Read the model definition and answer for the solid it produces. Units are mm, in the model's axes. Face numbers are marked on the shaded views. Round coordinates to 2 decimals unless told otherwise and drop trailing zeros. Order: outer loops, then holes, each group sorted by start corner. A loop starts at its lowest first (then second) coordinate and runs counter-clockwise, first axis right, second up.
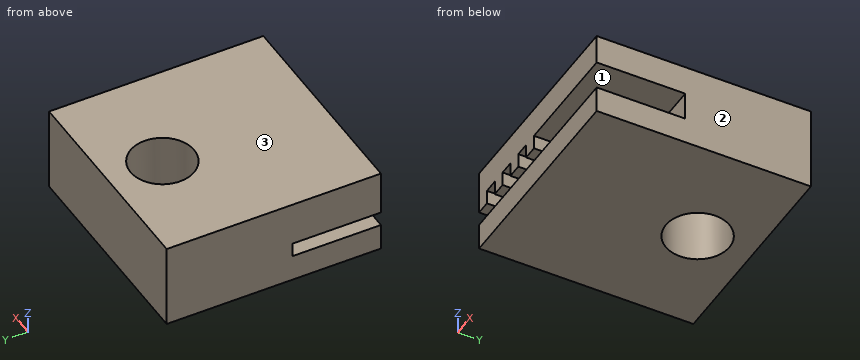
from build123d import *

# Parameters (mm, degrees)
F0_W     = 15
F0_H     = 15
F1_DEPTH = 6
F3_DEPTH = 6.2
F4_R     = 2.223391
F5_DEPTH = 25


with BuildPart() as f1:
    # F0 (on Top) → F1 (new body)
    with BuildSketch(Plane.XY):
        with Locations((13.635715, 2.612354)):
            Rectangle(F0_W, F0_H)
    extrude(amount=F1_DEPTH)

    # F2 (on face) → F3 (cut)
    with BuildSketch(Plane.XZ.offset(4.887646)):
        Polygon((6.135715, 2.883776), (6.135715, 1.883776), (21.135715, 1.883776), (21.135715, 3.883776), (14.135715, 3.883776), (13.135715, 3.883776), (13.135715, 2.883776), (12.135715, 2.883776), (12.135715, 3.883776), (11.135715, 3.883776), (11.135715, 2.883776), (10.135715, 2.883776), (10.135715, 3.883776), (9.135715, 3.883776), (9.135715, 2.883776), (8.135715, 2.883776), (8.135715, 3.883776), (7.135715, 3.883776), (7.135715, 2.883776), align=None)
    extrude(amount=-F3_DEPTH, mode=Mode.SUBTRACT)

    # F4 (on face) → F5 (cut)
    with BuildSketch(Plane(origin=(0, 0, 0), x_dir=(1, 0, 0), z_dir=(0, 0, -1))):
        with Locations((13.635715, -6.298021)):
            Circle(F4_R)
    extrude(amount=-F5_DEPTH, mode=Mode.SUBTRACT)


solid = f1.part
Q1. A cutting plane is placed at C-C, the plane z = 0.8. Give the vertices of the cut face in (x, y), plus the area to 3 significant figures.
Outcome:
outline: (6.14, -4.89) - (21.14, -4.89) - (21.14, 10.11) - (6.14, 10.11) - close; hole circle Ø4.45 at (13.64, 6.3)
area: 209 mm2
Q2. A cutting plane is placed at B-B, the plane x = 9.5. Give the vertices of the cut face in (y, z), plus the area to 3 significant figures.
Outcome:
outline: (-4.89, 0) - (10.11, 0) - (10.11, 6) - (-4.89, 6) - (-4.89, 3.88) - (1.31, 3.88) - (1.31, 1.88) - (-4.89, 1.88) - close
area: 77.6 mm2
Q3. A cutting plane is placed at A-A, the plane y = -1. Give the vertices of the cut face in (x, z).
Outcome:
outline: (6.14, 0) - (21.14, 0) - (21.14, 1.88) - (6.14, 1.88) - close; (6.14, 2.88) - (7.14, 2.88) - (7.14, 3.88) - (8.14, 3.88) - (8.14, 2.88) - (9.14, 2.88) - (9.14, 3.88) - (10.14, 3.88) - (10.14, 2.88) - (11.14, 2.88) - (11.14, 3.88) - (12.14, 3.88) - (12.14, 2.88) - (13.14, 2.88) - (13.14, 3.88) - (21.14, 3.88) - (21.14, 6) - (6.14, 6) - close
Q4. For a pull along Z with two mould halves and no side action, classify the marked faces 1, 2 and 3 as released by +Z, released by -Z, zero draft, split by the parting line, or undercut.
Outcome:
face 1: undercut
face 2: zero draft
face 3: released by +Z
Q5. A cutting plane is placed at D-D, the plane y = 7.75. Give the vertices of the cut face in (x, z), plus the area to 3 significant figures.
Outcome:
outline: (6.14, 0) - (11.95, 0) - (11.95, 6) - (6.14, 6) - close; (15.32, 0) - (21.14, 0) - (21.14, 6) - (15.32, 6) - close
area: 69.8 mm2
Q6. Flat-ended cylindrical pins translate along their axes: pin 1 (0.6 mm diameter, centred on x = 13.5, z = 3, fed in from -Y); pin 2 (2 mm diameter, centred on x = 9, y = -0.5, fed in from -Z); pin 3 (3.5 mm diameter, centred on x = 13.64, y = 6.3, fed in from -Z) (1 decimal); pin 4 (0.5 mm diameter, centred on y = -2.5, z = 3.5, fed in from +X). Find the tip coordinate at first contact, or state that the pin passes through.
Outcome:
pin 1: stops at y = 1.31
pin 2: stops at z = 0
pin 3: passes through
pin 4: stops at x = 13.14
Q7. Straight lines are drawn through the part: probe 1 along X at (y, z) = (-3, 3.05); probe 2 along Y at (x, z) = (13.5, 1.2); probe 3 along Y at (x, z) = (13.5, 2.15). For each, find the intervals that lie inside material, in ascending order.
Outcome:
probe 1: x = 6.14 to 7.14, 8.14 to 9.14, 10.14 to 11.14, 12.14 to 13.14
probe 2: y = -4.89 to 4.08, 8.52 to 10.11
probe 3: y = 1.31 to 4.08, 8.52 to 10.11
